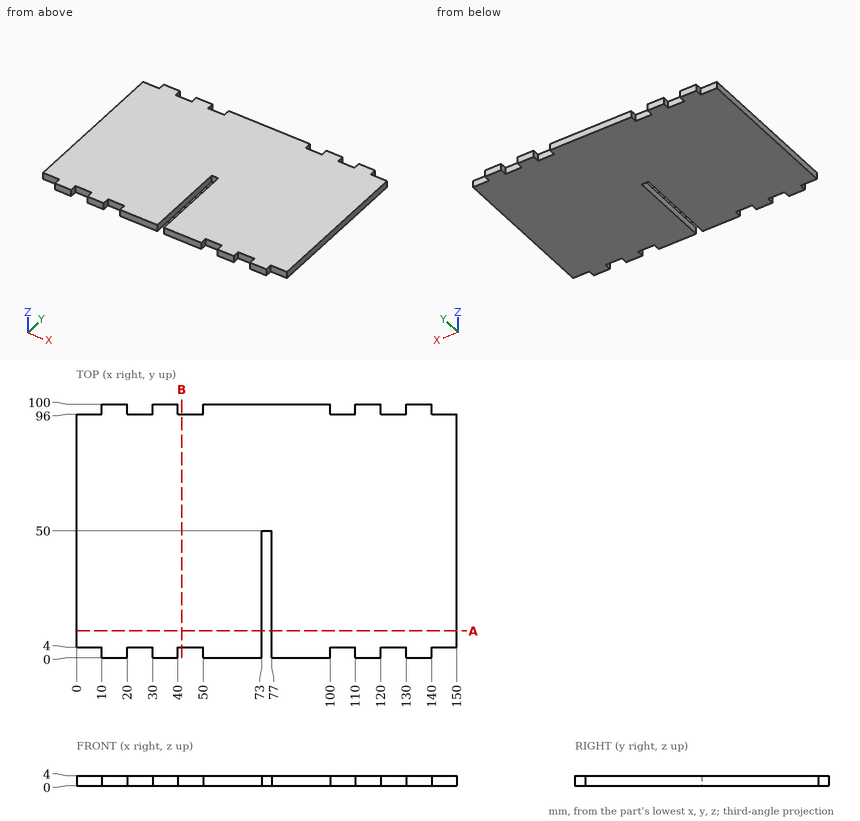
Geometry: see drawing. Coordinates: mm, zero at the bounding-box minimum. Give positions to 0.01 mm unless a question says otherwise; leave off trailing zeros. Loops run counter-clockwise (first coordinate to the right, second up) from the corner with the lowest first, then second, coordinate; pieces in that order, holes last. Notation, with made-up numbers: M 8,28.5 L 19,28.5 A9 cw 19,45.5 Z; hole C 72.5,17 d9. An arc over 180 degrees is marked long. Answer as CSV lines item,"result". Start each with the question number.
1. Line query: L1, parallel to X at y = 6, z = 2.3; L2, parallel to Y at x = 28, z = 3; L3, parallel to Y at x = 74.5, z = 2.65. Output: solid intervals per line, ascending.
2. Section B-B on x = 41.5. Return loops of the section in (y, z), plus the area to 3 significant figures.
3. Section A-A on y = 10.5. Return loops of the section in (x, z).
4. Pin query (flat end, axial travel): P1, Ø1.5, axis at x = 71, y = 48.5, coming from the -Z side; P2, Ø1, axis at x = 128.5, z = 2, coming from the +Y side; P3, Ø1.2, axis at x = 124.5, z = 2, coming from the -Y side; P4, Ø2, axis at y = 1, z = 1, coming from the +X side. Return the tip coordinate at first contact, or that it passes through.
Computed values:
1,L1,"x = 0 to 73, 77 to 150"
1,L2,"y = 4 to 96"
1,L3,"y = 50 to 100"
2,outline,"M 4,0 L 96,0 L 96,4 L 4,4 Z"
2,area,"368 mm²"
3,outline,"M 0,0 L 73,0 L 73,4 L 0,4 Z; M 77,0 L 150,0 L 150,4 L 77,4 Z"
4,P1,"stops at z = 0"
4,P2,"stops at y = 96"
4,P3,"stops at y = 4"
4,P4,"stops at x = 140"
